Source: CAD feature listing. Evaluate the final solid. Frame: model axes, mm. Face numbers are marked on the shaded views. Coordinates: 2 decimals unless noted, no trailing zeros. Loops run counter-clockwise (first coordinate to the right, second up) from the corner with the lowest first, then second, coordinate; pieces in that order, holes last.
Item 1: Section query A-A, the plane x = 0. Return the cut outline in (y, z), then the cut area to 3 significant figures.
Item 2: Line query: probe 1 along Y at (x, z) = (0, 53.75); probe 2 along X at (y, z) = (-25, 58.25); probe 3 along Y at (x, z) = (3, 59). Output: solid intervals per line, ascending.
Item 3: Pull-direction query (Y, two-part tool) for the marked faces 1, 2 and 3; classes: +Y half, -Y half, draft (parallel to the pull), parting line (faces both ways), or undercut.
Item 4: Pin query (flat end, axial travel): pin 1 Ø3 at (x, z) = (3, 57) entering from -Y; pin 2 Ø4 at (y, z) = (-21, 60) entering from -X; pin 3 Ø4 at (y, z) = (25, 54) entering from -X. Return the tip coordinate at first contact, or that it passes through.
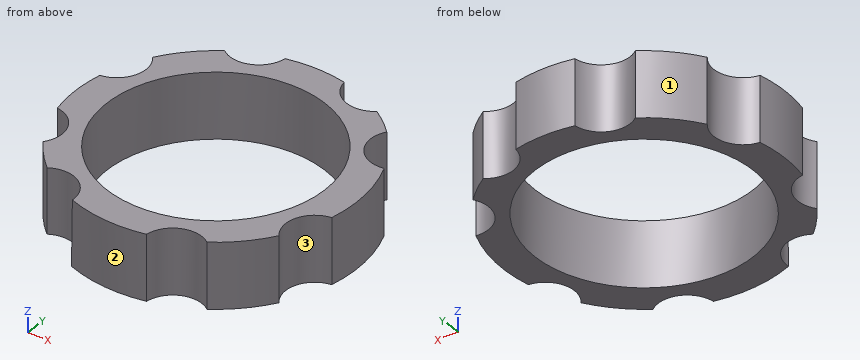
```python
from build123d import *

# Parameters (mm, degrees)
CYLINDER446_R               = 8
CYLINDER446_DEPTH           = 25
CYLINDER447_R               = 8
CYLINDER447_DEPTH           = 25
CYLINDER447_PLACEMENT_ANGLE = 225
CYLINDER448_R               = 8
CYLINDER448_DEPTH           = 25
CYLINDER449_R               = 8
CYLINDER449_DEPTH           = 25
CYLINDER449_ROLL_ANGLE      = -0.500355
CYLINDER449_PITCH_ANGLE     = 0.967193
CYLINDER449_PLACEMENT_ANGLE = 144.93646
CYLINDER450_R               = 8
CYLINDER450_DEPTH           = 25
CYLINDER451_R               = 8
CYLINDER451_DEPTH           = 25
CYLINDER451_PLACEMENT_ANGLE = 45
CYLINDER444_R               = 8
CYLINDER444_DEPTH           = 25
CYLINDER444_ROLL_ANGLE      = 0.146073
CYLINDER444_PITCH_ANGLE     = 1.079101
CYLINDER444_PLACEMENT_ANGLE = -9.939308
CYLINDER445_R               = 8
CYLINDER445_DEPTH           = 25
CYLINDER445_PLACEMENT_ANGLE = 45
TUBE023_R                   = 38.65
TUBE023_R_2                 = 30
TUBE023_DEPTH               = 18


with BuildPart() as obj1:
    # Cylinder446 → Cylinder446 (new body)
    with BuildSketch(Plane(origin=(-38.798949, 16.072537, 43), x_dir=(0, -1, 0), z_dir=(0, 0, 1))):
        Circle(CYLINDER446_R)
    extrude(amount=CYLINDER446_DEPTH)


with BuildPart() as obj2:
    # Cylinder447 → Cylinder447 (new body)
    with BuildSketch(Plane.XY):
        Circle(CYLINDER447_R)
    extrude(amount=CYLINDER447_DEPTH)


with BuildPart() as obj2_1:
    # Cylinder447 placement: moved
    add(obj2.part.moved(Location((-16.07, 38.8, 43))).rotate(Axis((-16.07, 38.8, 43), (0, 0, 1)), CYLINDER447_PLACEMENT_ANGLE))


with BuildPart() as obj3:
    # Cylinder448 → Cylinder448 (new body)
    with BuildSketch(Plane(origin=(16.072537, 38.798949, 43), x_dir=(-1, 0, 0), z_dir=(0, 0, 1))):
        Circle(CYLINDER448_R)
    extrude(amount=CYLINDER448_DEPTH)


with BuildPart() as obj4:
    # Cylinder449 → Cylinder449 (new body)
    with BuildSketch(Plane.XY):
        Circle(CYLINDER449_R)
    extrude(amount=CYLINDER449_DEPTH)


with BuildPart() as obj4_1:
    # Cylinder449 roll: moved
    add(obj4.part.rotate(Axis((0, 0, 0), (1, 0, 0)), CYLINDER449_ROLL_ANGLE))


with BuildPart() as obj4_2:
    # Cylinder449 pitch: moved
    add(obj4_1.part.rotate(Axis((0, 0, 0), (0, 1, 0)), CYLINDER449_PITCH_ANGLE))


with BuildPart() as obj4_3:
    # Cylinder449 placement: moved
    add(obj4_2.part.moved(Location((34.627801, 22.637113, 43.602309))).rotate(Axis((34.627801, 22.637113, 43.602309), (0, 0, 1)), CYLINDER449_PLACEMENT_ANGLE))


with BuildPart() as obj5:
    # Cylinder450 → Cylinder450 (new body)
    with BuildSketch(Plane(origin=(38.798949, -16.072537, 43), x_dir=(0, 1, 0), z_dir=(0, 0, 1))):
        Circle(CYLINDER450_R)
    extrude(amount=CYLINDER450_DEPTH)


with BuildPart() as obj6:
    # Cylinder451 → Cylinder451 (new body)
    with BuildSketch(Plane.XY):
        Circle(CYLINDER451_R)
    extrude(amount=CYLINDER451_DEPTH)


with BuildPart() as obj6_1:
    # Cylinder451 placement: moved
    add(obj6.part.moved(Location((16.07, -38.8, 43))).rotate(Axis((16.07, -38.8, 43), (0, 0, 1)), CYLINDER451_PLACEMENT_ANGLE))


with BuildPart() as obj7:
    # Cylinder444 → Cylinder444 (new body)
    with BuildSketch(Plane.XY):
        Circle(CYLINDER444_R)
    extrude(amount=CYLINDER444_DEPTH)


with BuildPart() as obj7_1:
    # Cylinder444 roll: moved
    add(obj7.part.rotate(Axis((0, 0, 0), (1, 0, 0)), CYLINDER444_ROLL_ANGLE))


with BuildPart() as obj7_2:
    # Cylinder444 pitch: moved
    add(obj7_1.part.rotate(Axis((0, 0, 0), (0, 1, 0)), CYLINDER444_PITCH_ANGLE))


with BuildPart() as obj7_3:
    # Cylinder444 placement: moved
    add(obj7_2.part.moved(Location((-21.748471, -35.690226, 43.196026))).rotate(Axis((-21.748471, -35.690226, 43.196026), (0, 0, 1)), CYLINDER444_PLACEMENT_ANGLE))


with BuildPart() as compound325:
    # Cylinder445 → Cylinder445 (new body)
    with BuildSketch(Plane.XY):
        Circle(CYLINDER445_R)
    extrude(amount=CYLINDER445_DEPTH)


with BuildPart() as compound325_1:
    # Cylinder445 placement: moved
    add(compound325.part.moved(Location((-38.8, -16.07, 43))).rotate(Axis((-38.8, -16.07, 43), (0, 0, -1)), CYLINDER445_PLACEMENT_ANGLE))

    # Compound325: union obj1, obj2, obj3, obj4, obj5, obj6, obj7
    add(obj1.part)
    add(obj2_1.part)
    add(obj3.part)
    add(obj4_3.part)
    add(obj5.part)
    add(obj6_1.part)
    add(obj7_3.part)


with BuildPart() as compound325_2:
    # Compound325 placement: moved
    add(compound325_1.part.moved(Location((0, 0, 3))))


with BuildPart() as cut:
    # Tube023 → Tube023 (new body)
    with BuildSketch(Plane.XY.offset(48)):
        Circle(TUBE023_R)
        Circle(TUBE023_R_2, mode=Mode.SUBTRACT)
    extrude(amount=TUBE023_DEPTH)

    # Cut: cut Compound325
    add(compound325_2.part, mode=Mode.SUBTRACT)


solid = cut.part
```
Verdict:
1. outline: (-38.65, 48) - (-30, 48) - (-30, 66) - (-38.65, 66) - close; (30, 48) - (38.65, 48) - (38.65, 66) - (30, 66) - close
1. area: 311 mm2
2. probe 1: y = -38.65 to -30, 30 to 38.65
2. probe 2: x = -29.48 to -16.58, 16.58 to 29.48
2. probe 3: y = -38.53 to -29.85, 29.85 to 38.53
3. face 1: +Y half
3. face 2: -Y half
3. face 3: undercut
4. pin 1: stops at y = -38.62
4. pin 2: stops at x = -32.47
4. pin 3: stops at x = -31.06
